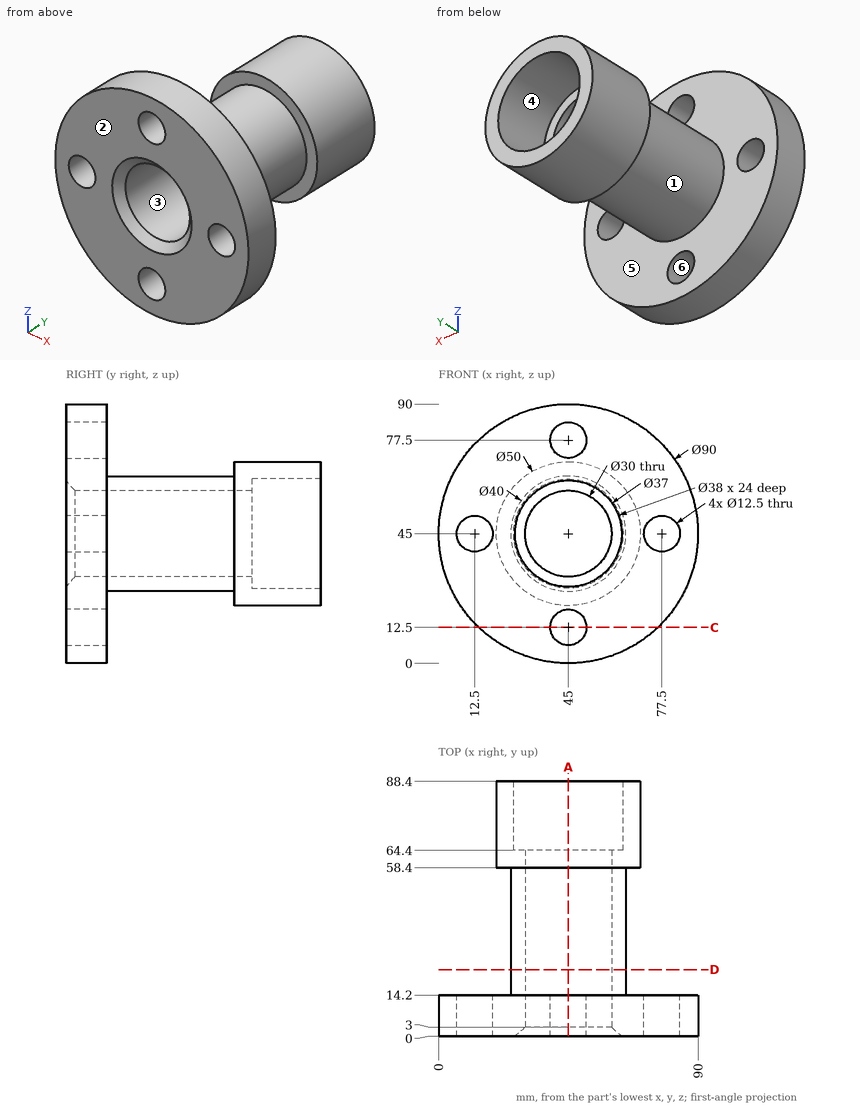
Source: three-view drawing plus pictorial views. Frame: mm from the lowest corner of the part. A direction names the side the tool comes from. Give positions to 0.01 mm unless a question says otherwise; leave off trailing zeros. Order: outer loops, then holes, each group sorted by start corner. A loop starts at its lowest first (then second) coordinate and runs counter-clockwise, first axis right, second up. Notation, with made-up numbers: (3, 80.25) - (61, 80.25) arc R17 ccw to (61, 90.25) - close; hole circle Ø4 at (36.5, 62). An arc over 180 degrees is marked (long way). Put each result on its own line as item: value.
Item 1: Draft query along Y for the marked faces 1, 2 and 3. Return one class per face: +Y half, -Y half, draft (parallel to the pull), parting line (faces both ways), or undercut.
Found:
face 1: undercut
face 2: -Y half
face 3: draft
Item 2: Ray query, L1, parallel to X at y = 5.25, z = 45; L2, parallel to Y at x = 62.5, z = 55.5; L3, parallel to X at y = 82.5, z = 45. Return the intervals inside material, ascending. Write a range as from..to.
Found:
L1: x = 0..6.25, 18.75..30, 60..71.25, 83.75..90
L2: y = 0..14.2, 58.4..88.4
L3: x = 20..26, 64..70
Item 3: Access query for the marked faces 4, 5 and 6. Directions: +Z, -Z, +X, -X, +Y, -Y. A direction counts if a zero-diameter tool reaches every point of the face in a straight line with its end or side. Return the directions, or none.
Found:
face 4: +Y
face 5: none
face 6: +Y, -Y
Item 4: Section query C-C, the plane z = 12.5. Return loops of the section in (x, y), then the cut area to 3 significant figures.
Found:
outline: (13.88, 0) - (38.75, 0) - (38.75, 14.2) - (13.88, 14.2) - close; (51.25, 0) - (76.12, 0) - (76.12, 14.2) - (51.25, 14.2) - close
area: 706 mm^2
Item 5: Contact query for flat-ended pins moving along their axis: pin 1 (12 mm diameter, centred on y = 21, z = 75.5, fed in from -X); pin 2 (3 mm diameter, centred on y = 39, z = 39.5, fed in from -X); pin 3 (5 mm diameter, centred on x = 51.5, y = 47.5, fed in from +Z); pin 4 (8 mm diameter, centred on x = 39, y = 72, fed in from -Z). Output: stop coordinate, or through.
Found:
pin 1: passes through
pin 2: stops at x = 25.4
pin 3: stops at z = 64.6
pin 4: stops at z = 20.08
Item 6: Section query A-A, the plane x = 45. Count the separate pieces of the cut face and the enclosed holes in it, then the cut area to 3 significant figures.
Found:
separate pieces: 4
enclosed holes: 0
area: 1,340 mm^2
Item 7: Section query D-D, the plane y = 23. Return loops of the section in (x, z).
Found:
outline: circle Ø40 at (45, 45); hole circle Ø30 at (45, 45)
